```python
from build123d import *

# Parameters (mm, degrees)
F0_W      = 105
F0_H      = 68
F1_DEPTH  = 30
F2_W      = 19.5
F2_H      = 43
F3_DEPTH  = 30.001
F4_R      = 16
F4_R_2    = 11
F5_DEPTH  = 19.5
F5_FACE_R = 11
F6_DEPTH  = 30.001


with BuildPart() as f1:
    # F0 (on Right) → F1 (new body)
    with BuildSketch(Plane.YZ):
        Rectangle(F0_W, F0_H)
    extrude(amount=F1_DEPTH)

    # F2 (on face) → F3 (cut, through all)
    with BuildSketch(Plane.YZ.offset(30)):
        with Locations((-42.75, 12.5)):
            Rectangle(F2_W, F2_H)
        with Locations((42.75, 12.5)):
            Rectangle(F2_W, F2_H)
    extrude(amount=-F3_DEPTH, mode=Mode.SUBTRACT)

    # F4 (on face) → F5 (cut)
    with BuildSketch(Plane.YZ.offset(30)):
        with Locations((0, 1)):
            Circle(F4_R)
        with Locations((0, 1)):
            Circle(F4_R_2, mode=Mode.SUBTRACT)
    extrude(amount=-F5_DEPTH, mode=Mode.SUBTRACT)

    # F5_face (on face) → F6 (cut, through all)
    with BuildSketch(Plane(origin=(30, 0, 1), x_dir=(0, 1, 0), z_dir=(1, 0, 0))):
        Circle(F5_FACE_R)
    extrude(amount=-F6_DEPTH, mode=Mode.SUBTRACT)


solid = f1.part
```
Geometry check sheet. Reference: the model listing, model coordinates, mm. A direction names the side the tool comes from. Coordinates: 2 decimals unless noted, no trailing zeros. Loops run counter-clockwise (first coordinate to the right, second up) from the corner with the lowest first, then second, coordinate; pieces in that order, holes last.
Item 1: Sectioned sample at C-C, the plane x = 15.5. Record the boundary of the cut face in (y, z), then the cut area to 3 significant figures.
Item 2: Release check for a two-part mould opening along Z. For faces 1 (the face through (15, -1, -34)), 2 (the face through (20.39, -3.47, -14.62)), 3 (the face through (15, 43, -9)) record: released by +Z, released by -Z, zero draft, split by the parting line, or undercut.
Item 3: Access from +Z, -Z, +X, -X, +Y, -Y to the whole of each face (thin tool, end or side, straight path). Record for faces 4 (the face through (15, 33, 12)), 5 (the face through (10.5, 3, 12)), 6 (the face through (30, 11, -15)), 7 (the face through (15, -33, 12)), 8 (the face through (15, -52.5, -22)).
Item 4: Sectioned sample at A-A, the plane y = 0. Record the boundary of the cut face in (x, z), then the cut area to 4 significant figures.
Item 5: Thickness scan on line 1 (Z direction, x = 20.75, y = 0); line 2 (Z direction, x = 7.25, y = 0); line 3 (Y direction, x = 18.5, z = 23). Record the ranges inside material, lowest first.
Item 6: Sectioned sample at D-D, the plane y = 14. Record the boundary of the cut face in (x, z).
Item 7: Go/stop test with flat-tipped pins: pin 1 Ø10 at (x, y) = (10.5, -43.5) entering from +Z; pin 2 Ø9 at (x, z) = (13, 15.5) entering from +Y; pin 3 Ø6 at (x, z) = (26.5, 13) entering from -Y. Record where each tip stops, or that it passes through.
Item 8: Sectioned sample at B-B, the plane z = -2. Record the boundary of the cut face in (x, y), then the cut area to 3 significant figures.
Check result:
1. outline: (-52.5, -34) - (52.5, -34) - (52.5, -9) - (33, -9) - (33, 34) - (-33, 34) - (-33, -9) - (-52.5, -9) - close; hole circle Ø32 at (0, 1)
1. area: 4,660 mm2
2. face 1: released by -Z
2. face 2: undercut
2. face 3: released by +Z
3. face 4: +Z, +X, -X, +Y
3. face 5: +X
3. face 6: +Z, -Z, +X, +Y, -Y
3. face 7: +Z, +X, -X, -Y
3. face 8: +Z, -Z, +X, -X, -Y
4. outline: (0, -34) - (30, -34) - (30, -15) - (10.5, -15) - (10.5, -10) - (0, -10) - close; (0, 12) - (10.5, 12) - (10.5, 17) - (30, 17) - (30, 34) - (0, 34) - close
4. area: 1,185 mm2
5. line 1: z = -34 to -15, 17 to 34
5. line 2: z = -34 to -10, 12 to 34
5. line 3: y = -33 to 33
6. outline: (0, -34) - (30, -34) - (30, -6.75) - (10.5, -6.75) - (10.5, 8.75) - (30, 8.75) - (30, 34) - (0, 34) - close
7. pin 1: stops at z = -9
7. pin 2: stops at y = 33
7. pin 3: stops at y = -33
8. outline: (0, -33) - (30, -33) - (30, -15.72) - (10.5, -15.72) - (10.5, -10.58) - (0, -10.58) - close; (0, 10.58) - (10.5, 10.58) - (10.5, 15.72) - (30, 15.72) - (30, 33) - (0, 33) - close
8. area: 1,140 mm2
